from build123d import *

# Parameters (mm, degrees)
SKETCH1_W                                       = 146
SKETCH1_H                                       = 71
BOSS_EXTRUDE1_DEPTH                             = 15
SHELL1_T                                        = -5
SKETCH2_W                                       = 5
SKETCH2_H                                       = 61
CUT_EXTRUDE1_DEPTH                              = 10
BOSS_EXTRUDE2_DEPTH                             = 10
CSK_FOR_M3_FLAT_HEAD_MACHINE_SCREW1_D           = 3.4
CSK_FOR_M3_FLAT_HEAD_MACHINE_SCREW1_DEPTH       = 10
CSK_FOR_M3_FLAT_HEAD_MACHINE_SCREW1_CSINK_D     = 6.3
CSK_FOR_M3_FLAT_HEAD_MACHINE_SCREW1_CSINK_ANGLE = 90
CSK_FOR_M3_FLAT_HEAD_MACHINE_SCREW1_TIP         = 1.021463052
FILLET1_R                                       = 3
CUT_EXTRUDE3_DEPTH                              = 10
FILLET2_R                                       = 2
SKETCH14_R                                      = 6
BOSS_EXTRUDE4_DEPTH                             = 5
F_3_5_3_5_DIAMETER_HOLE1_D                      = 3.5
CUT_EXTRUDE6_DEPTH                              = 2.5
CUT_EXTRUDE7_DEPTH                              = 10
CUT_EXTRUDE7_DEPTH_BACK                         = 1
SKETCH19_W                                      = 63
SKETCH19_H                                      = 38
CUT_EXTRUDE8_DEPTH                              = 83.54847061
FILLET4_R                                       = 2
FILLET5_R                                       = 3
F_3_3_3_3_DIAMETER_HOLE1_D                      = 3.3
SKETCH24_W                                      = 5.6
SKETCH24_H                                      = 2
CUT_EXTRUDE9_DEPTH                              = 5.6
SKETCH25_W                                      = 5.6
SKETCH25_H                                      = 2
CUT_EXTRUDE10_DEPTH                             = 5.6


with BuildPart() as part:
    # Sketch1 → Boss-Extrude1 (new body)
    with BuildSketch(Plane(origin=(0, 0, 0), x_dir=(1, 0, 0), z_dir=(0, 1, 0))):
        Rectangle(SKETCH1_W, SKETCH1_H)
    extrude(amount=BOSS_EXTRUDE1_DEPTH)

    # Shell1
    shell1_openings = [part.faces().sort_by_distance(p)[0] for p in [
        (0, 15, 0),
    ]]
    offset(amount=SHELL1_T, openings=shell1_openings, kind=Kind.INTERSECTION)

    # Sketch2 → Cut-Extrude1 (cut)
    with BuildSketch(Plane(origin=(0, 15, 0), x_dir=(1, 0, 0), z_dir=(0, 1, 0))):
        with Locations((-70.5, 0)):
            Rectangle(SKETCH2_W, SKETCH2_H)
    extrude(amount=-CUT_EXTRUDE1_DEPTH, mode=Mode.SUBTRACT)

    # Sketch3 → Boss-Extrude2 (add)
    with BuildSketch(Plane(origin=(0, 5, 0), x_dir=(1, 0, 0), z_dir=(0, 1, 0))):
        Polygon((-55.5, 23.5), (50.5, 23.5), (57.5, 30.5), (-62.5, 30.5), align=None)
        Polygon((-55.5, -23.5), (-62.5, -30.5), (57.5, -30.5), (50.5, -23.5), align=None)
    extrude(amount=BOSS_EXTRUDE2_DEPTH)

    # CSK for M3 Flat Head Machine Screw1
    with Locations(Plane(origin=(0, 0, 0), x_dir=(-1, 0, 0), z_dir=(0, -1, 0))):
        with Locations((-63, -27), (67, 27), (67, -27), (-63, 27)):
            CounterSinkHole(CSK_FOR_M3_FLAT_HEAD_MACHINE_SCREW1_D / 2, CSK_FOR_M3_FLAT_HEAD_MACHINE_SCREW1_CSINK_D / 2, depth=CSK_FOR_M3_FLAT_HEAD_MACHINE_SCREW1_DEPTH, counter_sink_angle=CSK_FOR_M3_FLAT_HEAD_MACHINE_SCREW1_CSINK_ANGLE)
            with Locations((0, 0, -(CSK_FOR_M3_FLAT_HEAD_MACHINE_SCREW1_DEPTH + CSK_FOR_M3_FLAT_HEAD_MACHINE_SCREW1_TIP / 2))):  # 118° drill point
                Cone(0, CSK_FOR_M3_FLAT_HEAD_MACHINE_SCREW1_D / 2, CSK_FOR_M3_FLAT_HEAD_MACHINE_SCREW1_TIP, mode=Mode.SUBTRACT)

    # Fillet1
    fillet1_edges = [part.edges().sort_by_distance(p)[0] for p in [
        (-73, 7.5, -35.5),
        (73, 7.5, -35.5),
        (73, 7.5, 35.5),
        (-73, 7.5, 35.5),
    ]]
    fillet(fillet1_edges, radius=FILLET1_R)

    # Sketch8 → Cut-Extrude3 (cut)
    with BuildSketch(Plane.XZ):
        Polygon((67.5, 0), (37.5, 23), (37.5, -23), align=None)
        Polygon((0, 4.383686057), (24.282148621, 23), (-24.282148621, 23), align=None)
        Polygon((2.5, 0), (32.5, -23), (32.5, 23), align=None)
        Polygon((-2.5, 0), (-32.5, 23), (-32.5, -23), align=None)
        Polygon((-67.5, 0), (-37.5, -23), (-37.5, 23), align=None)
        Polygon((-45.717851379, 23), (-67.5, 23), (-67.5, 6.300352724), align=None)
        Polygon((67.5, 6.300352724), (45.717851379, 23), (67.5, 23), align=None)
        Polygon((45.717851379, -23), (67.5, -23), (67.5, -6.300352724), align=None)
        Polygon((-67.5, -6.300352724), (-45.717851379, -23), (-67.5, -23), align=None)
        Polygon((-24.282148621, -23), (24.282148621, -23), (0, -4.383686057), align=None)
    extrude(amount=-CUT_EXTRUDE3_DEPTH, mode=Mode.SUBTRACT)

    # Fillet2
    fillet2_edges = [part.edges().sort_by_distance(p)[0] for p in [
        (-67.5, 2.5, 0),
        (-37.5, 2.5, 23),
        (-37.5, 2.5, -23),
        (0, 2.5, 4.383686057),
        (-24.282148621, 2.5, 23),
        (24.282148621, 2.5, 23),
        (45.717851379, 2.5, -23),
        (67.5, 2.5, -6.300352724),
        (67.5, 2.5, -23),
        (-67.5, 2.5, -23),
        (-67.5, 2.5, -6.300352724),
        (-45.717851379, 2.5, -23),
        (67.5, 2.5, 23),
        (67.5, 2.5, 6.300352724),
        (45.717851379, 2.5, 23),
        (-45.717851379, 2.5, 23),
        (-67.5, 2.5, 6.300352724),
        (-67.5, 2.5, 23),
        (-2.5, 2.5, 0),
        (-32.5, 2.5, -23),
        (-32.5, 2.5, 23),
        (2.5, 2.5, 0),
        (32.5, 2.5, 23),
        (32.5, 2.5, -23),
        (-24.282148621, 2.5, -23),
        (0, 2.5, -4.383686057),
        (24.282148621, 2.5, -23),
        (67.5, 2.5, 0),
        (37.5, 2.5, -23),
        (37.5, 2.5, 23),
    ]]
    fillet(fillet2_edges, radius=FILLET2_R)

    # Sketch14 → Boss-Extrude4 (add, through all)
    with BuildSketch(Plane(origin=(0, 5, 0), x_dir=(1, 0, 0), z_dir=(0, 1, 0))):
        with Locations((-35, 0)):
            Circle(SKETCH14_R)
    extrude(amount=-BOSS_EXTRUDE4_DEPTH)

    # Ø3.5 (3.5) Diameter Hole1 (through all)
    with Locations(Plane(origin=(0, 5, 0), x_dir=(1, 0, 0), z_dir=(0, 1, 0))):
        with Locations((-35, 0)):
            Hole(F_3_5_3_5_DIAMETER_HOLE1_D / 2)

    # Sketch17 → Cut-Extrude6 (cut)
    with BuildSketch(Plane(origin=(0, 5, 0), x_dir=(1, 0, 0), z_dir=(0, 1, 0))):
        Polygon((-31.766838493, 0), (-33.383419246, 2.8), (-36.616580754, 2.8), (-38.233161507, 0), (-36.616580754, -2.8), (-33.383419246, -2.8), align=None)
    extrude(amount=-CUT_EXTRUDE6_DEPTH, mode=Mode.SUBTRACT)

    # Sketch19 → Cut-Extrude7 (cut, two sides: drawn at the far end of the back side and taken through both)
    with BuildSketch(Plane.XZ.offset(-CUT_EXTRUDE7_DEPTH_BACK)):
        with Locations((-35, 0)):
            Rectangle(SKETCH19_W, SKETCH19_H)
    extrude(amount=CUT_EXTRUDE7_DEPTH + CUT_EXTRUDE7_DEPTH_BACK, mode=Mode.SUBTRACT)

    # Sketch20 → Cut-Extrude8 (cut, through all)
    with BuildSketch(Plane(origin=(0, 15, 0), x_dir=(1, 0, 0), z_dir=(0, 1, 0))):
        Polygon((-58.964466094, 34.035533906), (-60.428932188, 35.5), (55.428932188, 35.5), (53.964466094, 34.035533906), (48.428932188, 28.5), (-53.428932188, 28.5), align=None)
        Polygon((-58.964466094, -34.035533906), (-53.428932188, -28.5), (48.428932188, -28.5), (53.964466094, -34.035533906), (55.428932188, -35.5), (-60.428932188, -35.5), align=None)
    extrude(amount=-CUT_EXTRUDE8_DEPTH, mode=Mode.SUBTRACT)

    # Fillet4
    fillet4_edges = [part.edges().sort_by_distance(p)[0] for p in [
        (-73, 10, -30.5),
        (-73, 10, 30.5),
    ]]
    fillet(fillet4_edges, radius=FILLET4_R - 0.0001)  # a hair under: the kernel refuses the full size

    # Fillet5
    fillet5_edges = [part.edges().sort_by_distance(p)[0] for p in [
        (68, 10, 30.5),
        (68, 10, -30.5),
        (-62.5, 10, -30.5),
        (-62.5, 10, 30.5),
    ]]
    fillet(fillet5_edges, radius=FILLET5_R)

    # Ø3.3 (3.3) Diameter Hole1 (through all)
    with Locations(Plane(origin=(0, 0, 0), x_dir=(-1, 0, 0), z_dir=(0, -1, 0))):
        with Locations((-23, 26), (-23, -26)):
            Hole(F_3_3_3_3_DIAMETER_HOLE1_D / 2)

    # Sketch24 → Cut-Extrude9 (cut)
    with BuildSketch(Plane.XY.offset(28.5)):
        with Locations((23, 4)):
            Rectangle(SKETCH24_W, SKETCH24_H)
    extrude(amount=-CUT_EXTRUDE9_DEPTH, mode=Mode.SUBTRACT)

    # Sketch25 → Cut-Extrude10 (cut)
    with BuildSketch(Plane(origin=(0, 0, -28.5), x_dir=(-1, 0, 0), z_dir=(0, 0, -1))):
        with Locations((-23, 4)):
            Rectangle(SKETCH25_W, SKETCH25_H)
    extrude(amount=-CUT_EXTRUDE10_DEPTH, mode=Mode.SUBTRACT)


solid = part.part
Geometry check sheet. Reference: the model listing, model coordinates, mm. A direction names the side the tool comes from. Give positions to 0.01 mm unless a question says otherwise; leave off trailing zeros. Use a Markdown table: item, result.
Item 1: Material ranges on line 1 along Z through (x, y) = (23, 8.25); line 2 along X through (y, z) = (4.25, 27); line 3 along Z through (x, y) = (9.5, 8), recorded low to high.
Answers follow:
| item | result |
|---|---|
| line 1 | z = -28.5 to -27.65, -24.35 to -23.5, 23.5 to 24.35, 27.65 to 28.5 |
| line 2 | x = -73 to -68.7, -65.3 to 20.2, 25.8 to 61.3, 64.7 to 73 |
| line 3 | z = -28.5 to -23.5, 23.5 to 28.5 |
Item 2: Draft check along Z on faces 5 (the flat face through (57.437, 2.465, 14.015)), 6 (the flat face through (-2, 8, -28.5)), 7 (the flat face through (-73, 2, 0)). Enter one of: +Z half, -Z half, draft (parallel to the pull), parting line (faces both ways), or undercut.
Answers follow:
| item | result |
|---|---|
| face 5 | undercut |
| face 6 | -Z half |
| face 7 | draft |
Item 3: Section check A-A (z = 16.5). State how many separate pieces and enclosed holes the cut face has, and give its area (3 significant figures).
Answers follow:
| item | result |
|---|---|
| separate pieces | 8 |
| enclosed holes | 0 |
| area | 298 mm2 |
Item 4: Tool access check on faces 1 (the flat face through (-32.586, 3.768, 1.42)), 2 (the flat face through (-67, 10, -30.5)), 3 (the cylindrical face through (-38.64, 2.54, 20.75)), 4 (the cylindrical face through (-72.14, 7.6, -34.6)). Record the directions out of +Z, -Z, +X, -X, +Y, -Y that give a thin tool (end or side, any length) a straight path to the whole face; none if there is none.
Answers follow:
| item | result |
|---|---|
| face 1 | +Y |
| face 2 | -X, +Y |
| face 3 | +Y, -Y |
| face 4 | -Z, -X, +Y, -Y |
Item 5: Depth check by flat-ended pin: P1, Ø1.5, axis at x = 35, y = 13, coming from the -Z side; P2, Ø3, axis at x = -34, z = -0.5, coming from the +Y side; P3, Ø12, axis at x = 7.5, z = -12.5, coming from the +Y side; P4, Ø4.5, axis at x = 23, z = 26, coming from the +Y side. Enter the tip coordinate at first touch or a pass-through.
Answers follow:
| item | result |
|---|---|
| P1 | stops at z = -28.5 |
| P2 | stops at y = 2.5 |
| P3 | stops at y = 5 |
| P4 | stops at y = 15 |
